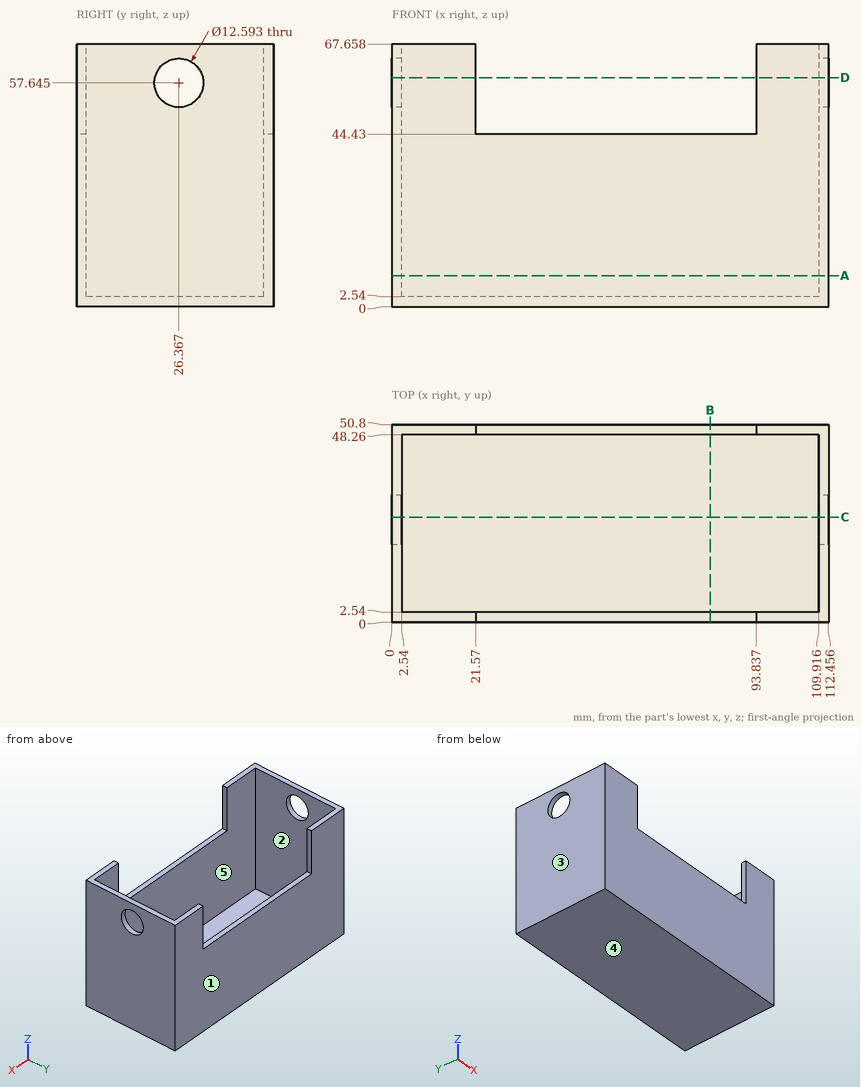
Check sheet for the drawn part. Datum: minimum x, y, z corner. Units: mm. A direction names the side the tool comes from. Give positions to 0.01 mm unless a question says otherwise; leave off trailing zeros. Write each loop counter-clockwise with the first axis right and the second up, starting at its lowest first coordinate (ties: lowest second). Pieces come first, ordered by that corner, then holes.
(1) Material ranges on line 1 (Y direction, x = 93, z = 14); line 2 (X direction, y = 30.5, z = 51); line 3 (Z direction, x = 47, y = 29.5), recorded low to high.
(2) Access from +Z, -Z, +X, -X, +Y, -Y to the whole of each face (thin tool, end or side, straight path). Record for the marked faces 4 and 5.
(3) Cross-section at B-B (x = 82). Enter the section's corners in (y, z), plus the area to 3 significant figures.
(4) Cross-section at C-C (y = 27). Enter the section's corners in (x, z).
(5) Cross-section at D-D (z = 59). Enter the section's corners in (x, y).
(6) Cross-section at A-A (z = 8). Enter the section's corners in (x, y).
(7) Gauge pin test, flat ends, axial feed: pin 1 (3 mm diameter, centred on x = 88, y = 29.5, fed in from +Z); pin 2 (1.3 mm diameter, centred on x = 48.5, y = 0.5, fed in from +Z). Record the tip position at first contact, or that the pin passes through.
(8) Mould release check, pull along X, two halves, no side actions. Record for the marked faces 1, 2 and 3: +X half, -X half, draft (parallel to the pull), parting line (faces both ways), or undercut.
Worked out:
1. line 1: y = 0 to 2.54, 48.26 to 50.8
1. line 2: x = 0 to 2.54, 109.92 to 112.46
1. line 3: z = 0 to 2.54
2. face 4: -Z, +X, -X, +Y, -Y
2. face 5: +Z
3. outline: (0, 0) - (50.8, 0) - (50.8, 44.43) - (48.26, 44.43) - (48.26, 2.54) - (2.54, 2.54) - (2.54, 44.43) - (0, 44.43) - close
3. area: 342 mm2
4. outline: (0, 0) - (112.46, 0) - (112.46, 51.38) - (109.92, 51.38) - (109.92, 2.54) - (2.54, 2.54) - (2.54, 51.38) - (0, 51.38) - close; (0, 63.91) - (2.54, 63.91) - (2.54, 67.66) - (0, 67.66) - close; (109.92, 63.91) - (112.46, 63.91) - (112.46, 67.66) - (109.92, 67.66) - close
5. outline: (0, 0) - (21.57, 0) - (21.57, 2.54) - (2.54, 2.54) - (2.54, 20.22) - (0, 20.22) - close; (0, 32.52) - (2.54, 32.52) - (2.54, 48.26) - (21.57, 48.26) - (21.57, 50.8) - (0, 50.8) - close; (93.84, 0) - (112.46, 0) - (112.46, 20.22) - (109.92, 20.22) - (109.92, 2.54) - (93.84, 2.54) - close; (93.84, 48.26) - (109.92, 48.26) - (109.92, 32.52) - (112.46, 32.52) - (112.46, 50.8) - (93.84, 50.8) - close
6. outline: (0, 0) - (112.46, 0) - (112.46, 50.8) - (0, 50.8) - close; hole (2.54, 2.54) - (109.92, 2.54) - (109.92, 48.26) - (2.54, 48.26) - close
7. pin 1: stops at z = 2.54
7. pin 2: stops at z = 44.43
8. face 1: draft
8. face 2: undercut
8. face 3: -X half
